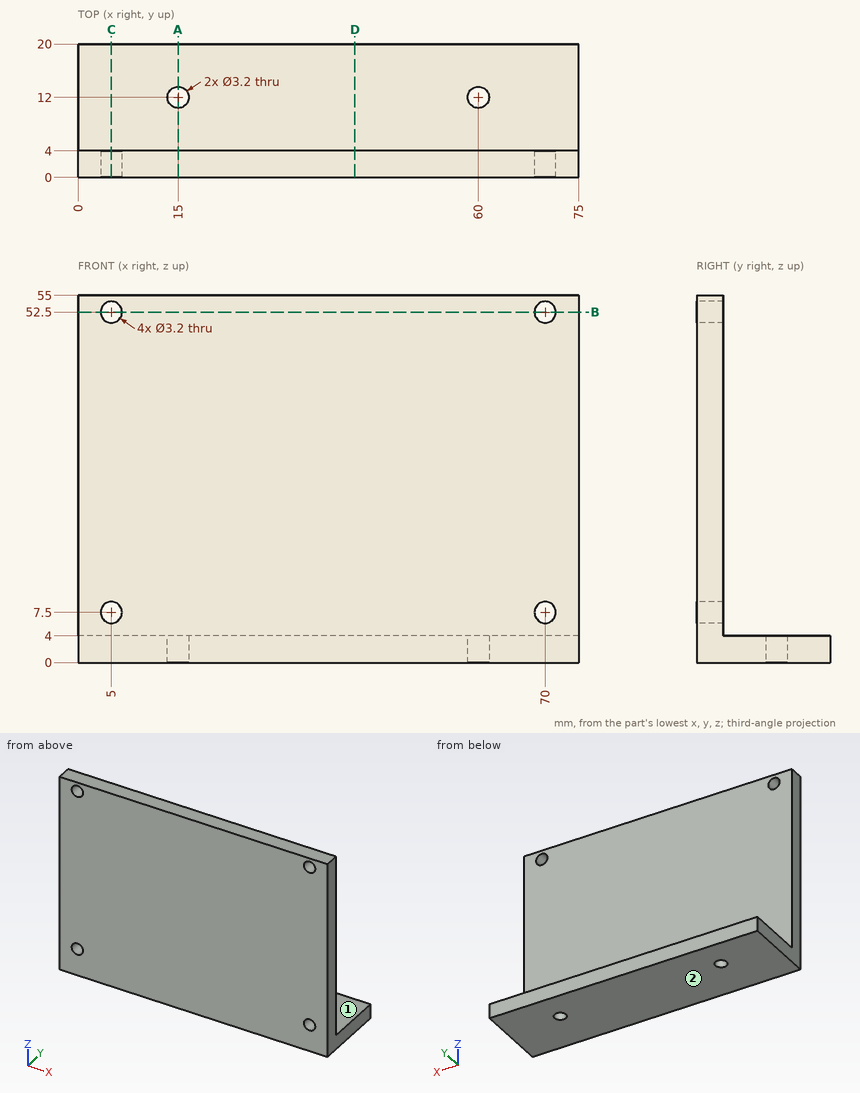
Part print with two shaded views. Sizes in mm from the minimum x, y, z corner. A direction names the side the tool comes from. Coordinates: 2 decimals unless noted, no trailing zeros. Order: outer loops, then holes, each group sorted by start corner. A loop starts at its lowest first (then second) coordinate and runs counter-clockwise, first axis right, second up. Notation, with made-up numbers: (42, 19.25) - (48, 19.25) arc R33 ccw to (48, 57.25) - close; hole circle Ø4 at (-13, 73.25). An arc over 180 degrees is marked (long way). Answer in a Markdown table with one row per item.
1. 3-axis set-ups, long thin cutter, end or side, ignore diameter. For the marked faces 1 and 2: which of +Z, -Z, +X, -X, +Y, -Y reach the whole face in a straight line?
Answer:
| item | result |
|---|---|
| face 1 | +Z, +X, -X, +Y |
| face 2 | -Z, +X, -X, +Y, -Y |
2. Drill centre lines: L1, parallel to Z at x = 70, y = 2.9; L2, parallel to Z at x = 26.5, y = 19. Where is each one in solid material? Low to high. Write a range as from..to.
Answer:
| item | result |
|---|---|
| L1 | 0..5.9, 9.1..50.9, 54.1..55 |
| L2 | 0..4 |
3. Slice it at C-C, the plane x = 5. List the corners of the cut face in (y, z).
Answer:
| item | result |
|---|---|
| outline | (0, 0) - (20, 0) - (20, 4) - (4, 4) - (4, 5.9) - (0, 5.9) - close; (0, 9.1) - (4, 9.1) - (4, 50.9) - (0, 50.9) - close; (0, 54.1) - (4, 54.1) - (4, 55) - (0, 55) - close |
4. Flat gauge pins, fed straight in: P1, Ø2.5, axis at x = 5, z = 7.5, coming from the +Y side; P2, Ø3, axis at x = 16, z = 14.5, coming from the +Y side; P3, Ø5, axis at x = 20, y = 14.5, coming from the +Z side. Where does each tip first touch, or does it go through?
Answer:
| item | result |
|---|---|
| P1 | through |
| P2 | y = 4 |
| P3 | z = 4 |
5. Slice it at D-D, the plane x = 41.5. List the corners of the cut face in (y, z).
Answer:
| item | result |
|---|---|
| outline | (0, 0) - (20, 0) - (20, 4) - (4, 4) - (4, 55) - (0, 55) - close |
6. Slice it at A-A, the plane x = 15. List the corners of the cut face in (y, z).
Answer:
| item | result |
|---|---|
| outline | (0, 0) - (10.4, 0) - (10.4, 4) - (4, 4) - (4, 55) - (0, 55) - close; (13.6, 0) - (20, 0) - (20, 4) - (13.6, 4) - close |
7. Slice it at B-B, the plane z = 52.5. List the corners of the cut face in (x, y), then the cut area to 3 significant figures.
Answer:
| item | result |
|---|---|
| outline | (0, 0) - (3.4, 0) - (3.4, 4) - (0, 4) - close; (6.6, 0) - (68.4, 0) - (68.4, 4) - (6.6, 4) - close; (71.6, 0) - (75, 0) - (75, 4) - (71.6, 4) - close |
| area | 274 mm² |
